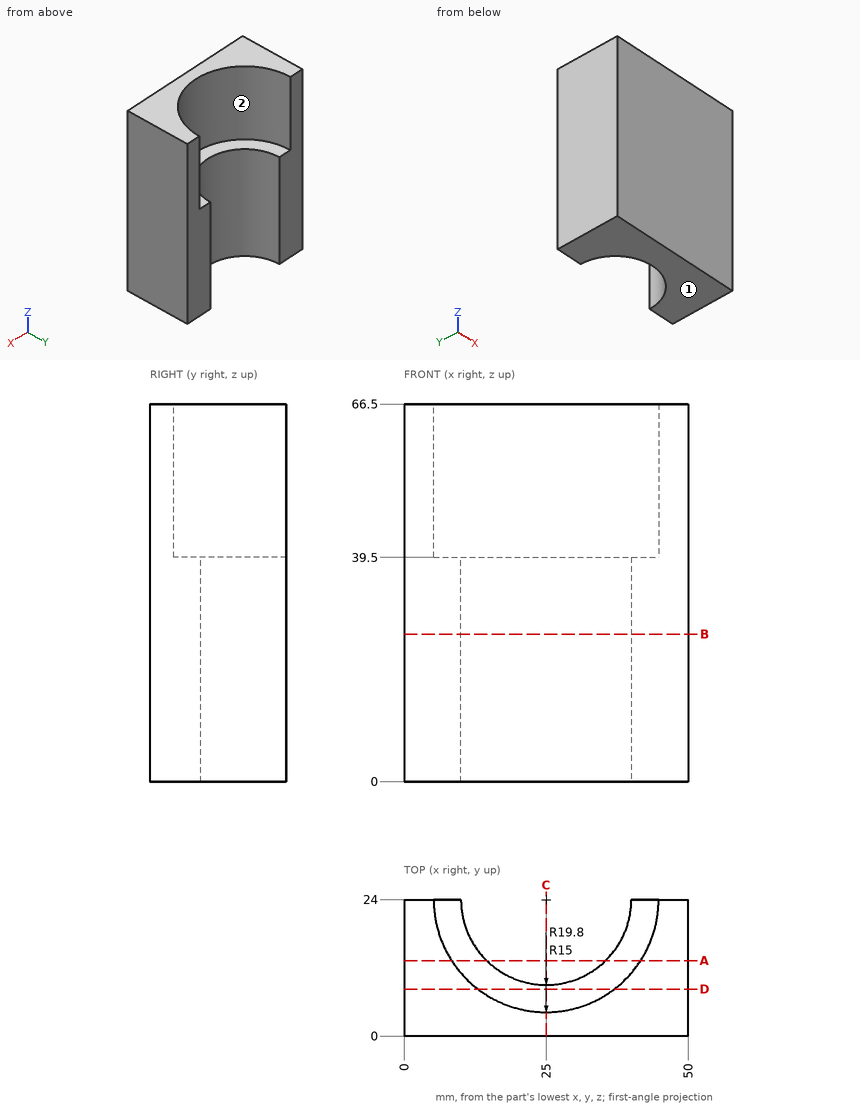
Drawing for the job (mm, zero at the part's lowest x, y, z). A direction names the side the tool comes from. Coordinates: 2 decimals unless noted, no trailing zeros. Write each loop counter-clockwise with the first axis right and the second up, starting at its lowest first coordinate (ties: lowest second). Pieces come first, ordered by that corner, then holes. Notation, with made-up numbers: (9.25, 14.5) - (50.25, 14.5) arc R10 cw to (50.25, 32.5) - close; hole circle Ø7 at (57, -12). An arc over 180 degrees is marked (long way). Write each question's results on one line, items separated by ' | '. Start each with the question number.
1) Cut at A-A (y = 13.25). Write the cut outline in (x, z).
2) Cut at B-B (z = 26). Write the cut outline in (x, y).
3) Flat gauge pins, fed straight in: P1, Ø5, axis at x = 17.5, y = 11.5, coming from the +Z side; P2, Ø1.5, axis at x = 23.5, y = 10.5, coming from the +Z side; P3, Ø8, axis at x = 29, z = 47.5, coming from the +Y side. Where does each tip first touch, or does it go through?
4) Cut at C-C (x = 25). Write the cut outline in (y, z), then the cut area to 3 significant figures.
5) 3-axis set-ups, long thin cutter, end or side, ignore diameter. For the marked faces 1 and 2: which of +Z, -Z, +X, -X, +Y, -Y reach the whole face in a straight line?
6) Probe line 1 along X through (y, z) = (21.5, 45); line 2 along Y through (x, z) = (25, 5.5); line 3 along X through (y, z) = (14, 30). List the from-to ranges inside material, lowest first. Write a range as from..to.
7) Cut at D-D (y = 8.25). Write the cut outline in (x, z).
Returned:
1) outline: (0, 0) - (14.54, 0) - (14.54, 39.5) - (8.37, 39.5) - (8.37, 66.5) - (0, 66.5) - close; (35.46, 0) - (50, 0) - (50, 66.5) - (41.63, 66.5) - (41.63, 39.5) - (35.46, 39.5) - close
2) outline: (0, 0) - (50, 0) - (50, 24) - (40, 24) arc R15 cw to (10, 24) - (0, 24) - close
3) P1: z = 39.5 | P2: through | P3: y = 5.89
4) outline: (0, 0) - (9, 0) - (9, 39.5) - (4.2, 39.5) - (4.2, 66.5) - (0, 66.5) - close | area: 469 mm^2
5) face 1: -Z, +X, -X, +Y, -Y | face 2: +Z, +Y
6) line 1: 0..5.36, 44.64..50 | line 2: 0..9 | line 3: 0..13.82, 36.18..50
7) outline: (0, 0) - (50, 0) - (50, 66.5) - (37, 66.5) - (37, 39.5) - (13, 39.5) - (13, 66.5) - (0, 66.5) - close
